from build123d import *

# Parameters (mm, degrees)
SKETCH2_R               = 10
BOSS_EXTRUDE1_DEPTH     = 25
SKETCH3_R               = 3
CUT_EXTRUDE1_DEPTH      = 11
CUT_EXTRUDE1_DEPTH_BACK = 20
SKETCH4_R               = 2.65
CUT_EXTRUDE2_DEPTH      = 21
SKETCH5_R               = 14
CUT_EXTRUDE3_DEPTH      = 2.5
FILLET1_R               = 0.5
CHAMFER1_SIZE           = 0.25
FILLET2_R               = 0.5


with BuildPart() as part:
    # Sketch2 → Boss-Extrude1 (new body, symmetric)
    with BuildSketch(Plane.XY):
        Polygon((7, 0), (-7, 0), (-13, 6), (-26, 6), (-26, 30), (-27, 31), (-27, 40), (-26, 41), (-14, 41), (-13, 40), (13, 40), (14, 41), (26, 41), (27, 40), (27, 31), (26, 30), (26, 6), (13, 6), align=None)
        with Locations((0, 20)):
            Circle(SKETCH2_R, mode=Mode.SUBTRACT)
    extrude(amount=BOSS_EXTRUDE1_DEPTH, both=True)

    # Sketch3 → Cut-Extrude1 (cut, two sides)
    with BuildSketch(Plane(origin=(0, 40, 0), x_dir=(1, 0, 0), z_dir=(0, 1, 0))) as cut_extrude1_sk:
        with Locations((20, -20)):
            Circle(SKETCH3_R)
        with Locations((20, 20)):
            Circle(SKETCH3_R)
        with Locations((-20, -20)):
            Circle(SKETCH3_R)
        with Locations((-20, 20)):
            Circle(SKETCH3_R)
    extrude(amount=CUT_EXTRUDE1_DEPTH, mode=Mode.SUBTRACT)
    extrude(cut_extrude1_sk.sketch, amount=-CUT_EXTRUDE1_DEPTH_BACK, mode=Mode.SUBTRACT)

    # Sketch4 → Cut-Extrude2 (cut, through all)
    with BuildSketch(Plane(origin=(0, 20, 0), x_dir=(1, 0, 0), z_dir=(0, 1, 0))):
        with Locations((-20, -20)):
            Circle(SKETCH4_R)
        with Locations((20, -20)):
            Circle(SKETCH4_R)
        with Locations((20, 20)):
            Circle(SKETCH4_R)
        with Locations((-20, 20)):
            Circle(SKETCH4_R)
    extrude(amount=-CUT_EXTRUDE2_DEPTH, mode=Mode.SUBTRACT)

    # Sketch5 → Cut-Extrude3 (cut)
    with BuildSketch(Plane.XY.offset(25)):
        with Locations((0, 20)):
            Circle(SKETCH5_R)
    cut_extrude3 = extrude(amount=-CUT_EXTRUDE3_DEPTH, mode=Mode.SUBTRACT)

    # Mirror1: Cut-Extrude3 across plane
    add(cut_extrude3.mirror(Plane.XY), mode=Mode.SUBTRACT)

    # Fillet1
    fillet1_edges = [part.edges().sort_by_distance(p)[0] for p in [
        (7, 0, 0),
        (-7, 0, 0),
        (-13, 6, 0),
        (-26, 30, 0),
        (-27, 31, 0),
        (-13, 40, 0),
        (13, 40, 0),
        (26, 30, 0),
        (13, 6, 0),
        (-10, 20, -22.5),
    ]]
    fillet(fillet1_edges, radius=FILLET1_R)

    # Chamfer1
    chamfer1_edges = [part.edges().sort_by_distance(p)[0] for p in [
        (-26, 6, 0),
        (26, 6, 0),
    ]]
    chamfer(chamfer1_edges, length=CHAMFER1_SIZE)

    # Fillet2
    fillet2_edges = [part.edges().sort_by_distance(p)[0] for p in [
        (-14, 20, 25),
        (-14, 20, -25),
    ]]
    fillet(fillet2_edges, radius=FILLET2_R)


solid = part.part
Geometry: final body of the model. Coordinates: model frame, mm. A direction names the side the tool comes from. Give positions to 0.01 mm unless a question says otherwise; leave off trailing zeros. Write each loop counter-clockwise with the first axis right and the second up, starting at its lowest first coordinate (ties: lowest second). Pieces come first, ordered by that corner, then holes. Notation, with made-up numbers: M 15.5,42 L 26.5,42 A35 ccw 26.5,80 Z; hole C 14.25,68.5 d2. An arc over 180 degrees is marked long. Answer in a Markdown table with one row per item. Add a question column.
(1) Ray query, line 1 (Z direction, x = -20, y = 29); line 2 (X direction, y = 34, z = 20); line 3 (Z direction, x = 20, y = 10). Return the intervals inside material, ascending.
(2) Section B-B on z = 20. State how many separate pieces and enclosed holes the cut face has, and give its area (3 significant figures).
(3) First-contact query: pin 1 (7 mm diameter, centred on y = 16.5, z = -11.5, fed in from +X); pin 2 (19 mm diameter, centred on y = 14.5, z = 1.5, fed in from -X); pin 3 (10 mm diameter, centred on x = 22, z = 8, fed in from -Y). Flat tips, straight axial feed; report the tip coordinate or a pass-through.
(4) Mould query, pull axis Y, two halves, no side actions, for faces 6 (the flat face through (-3, 30, 22.5)), 7 (the cylindrical face through (17.6, 30.4, -18.2)), 8 (the cylindrical face through (6.5, 7.6, -23.5)), 9 (the flat face through (0, 0, 0)). Classes: +Y half, -Y half, draft (parallel to the pull), parting line (faces both ways), or undercut.
(5) Section A-A on x = -20. Return loops of the section in (y, z).
(6) Reachability of faces 1 (the flat face through (-26, 18, 0)), 2 (the cylindrical face through (-17.472, 13.098, -20.796)), 3 (the cylindrical face through (-22.4, 30.4, 21.8)), 4 (the cylindrical face through (6.5, 7.6, 23.5)), 5 (the flat face through (20, 6, 0)) from +Z, -Z, +X, -X, +Y, -Y: full face, straight path, thin tool, end or side. Return the list, or none.
Result set:
| question | item | result |
|---|---|---|
| 1 | line 1 | z = -25 to -23, -17 to 17, 23 to 25 |
| 1 | line 2 | x = -27 to -23, -17 to 17, 23 to 27 |
| 1 | line 3 | z = -25 to -22.65, -17.35 to 17.35, 22.65 to 25 |
| 2 | separate pieces | 3 |
| 2 | enclosed holes | 1 |
| 2 | area | 1,220 mm^2 |
| 3 | pin 1 | stops at x = 26 |
| 3 | pin 2 | stops at x = -26 |
| 3 | pin 3 | stops at y = 6 |
| 4 | face 6 | undercut |
| 4 | face 7 | draft |
| 4 | face 8 | undercut |
| 4 | face 9 | -Y half |
| 5 | outline | M 6,-25 L 41,-25 L 41,-23 L 20,-23 L 20,-22.65 L 6,-22.65 Z; M 6,-17.35 L 20,-17.35 L 20,-17 L 41,-17 L 41,17 L 20,17 L 20,17.35 L 6,17.35 Z; M 6,22.65 L 20,22.65 L 20,23 L 41,23 L 41,25 L 6,25 Z |
| 6 | face 1 | +Z, -Z, -X, -Y |
| 6 | face 2 | +Y, -Y |
| 6 | face 3 | +Y |
| 6 | face 4 | +Z |
| 6 | face 5 | +Z, -Z, +X, -Y |
